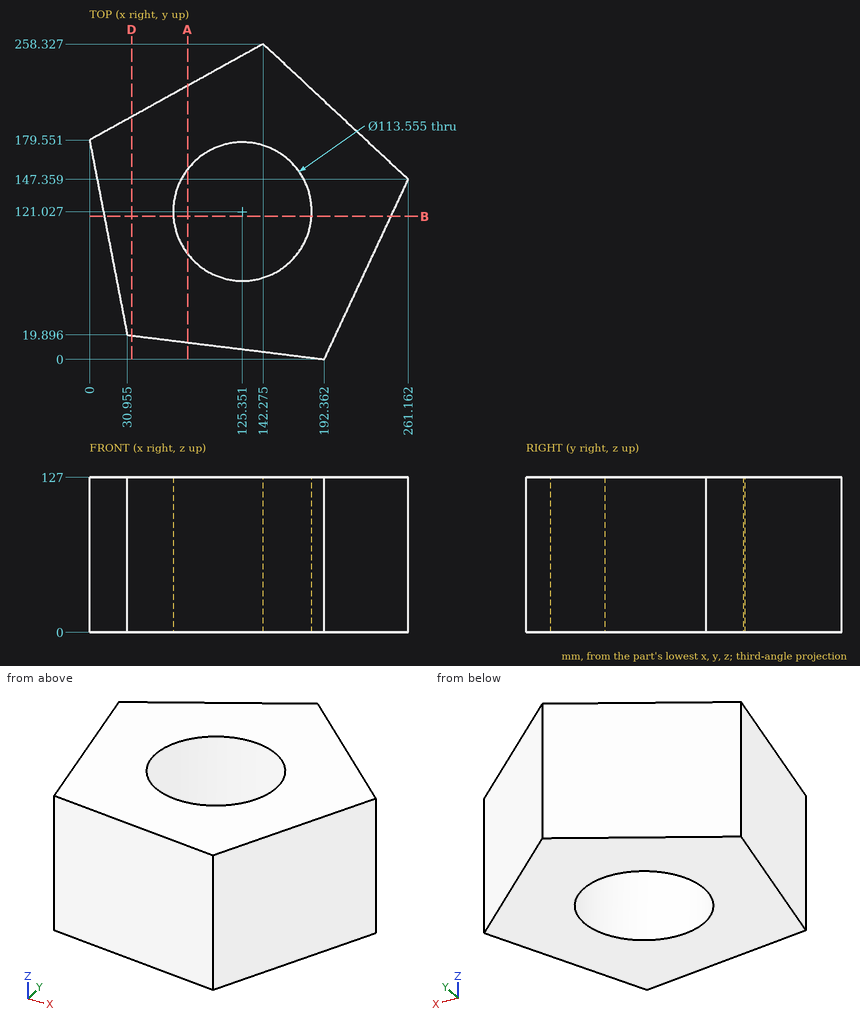
The figure shows three views and two pictorial views of one solid part (mm, origin at its lowest corner). Answer the questions. Give positions to 0.01 mm unless a question says otherwise; leave off trailing zeros. Order: outer loops, then holes, each group sorted by start corner. A loop starts at its lowest first (then second) coordinate and runs counter-clockwise, first axis right, second up. Notation, with made-up numbers: (28.25, 73.5) -> (38.25, 73.5) arc R8 ccw to (38.25, 84.5) -> close; hole circle Ø6 at (19, -24). An arc over 180 degrees is marked (long way). Answer as CSV lines item,"result". Start each with the question number.
Q1. A cutting plane is placed at D-D (x = 34.5). Determine the outline of the cut face in (y, z).
Q2. A cutting plane is placed at A-A (x = 80.5). Determine the outline of the cut face in (y, z).
Q3. Find the intervals of material crossed by L1, parallel to Y at x = 103, z = 109 (1 decimal); L2, parallel to Y at x = 76.5, z = 74 (1 decimal); L3, parallel to X at y = 110, z = 74 (1 decimal), in increasing order.
Q4. Given pin 1 (1 mm diameter, centred on x = 66.5, z = 43.5, fed in from +Y); pin 2 (8 mm diameter, centred on y = 93.5, z = 100, fed in from -X); pin 3 (6 mm diameter, centred on y = 100, z = 98.5, fed in from +X), each flat-ended and moving along its own axis, determine where each tip first touches the part or whether it passes through.
Q5. A cutting plane is placed at B-B (y = 117). Determine the outline of the cut face in (x, z) (1 decimal), then the cut area to 3 significant figures.
Results found:
1,outline,"(19.46, 0) -> (198.65, 0) -> (198.65, 127) -> (19.46, 127) -> close"
2,outline,"(13.79, 0) -> (86.21, 0) -> (86.21, 127) -> (13.79, 127) -> close; (155.84, 0) -> (224.12, 0) -> (224.12, 127) -> (155.84, 127) -> close"
3,L1,"11 to 68.8, 173.2 to 236.6"
3,L2,"14.3 to 92.1, 150 to 221.9"
3,L3,"13.5 to 69.7, 181 to 243.7"
4,pin 1,"y = 216.65"
4,pin 2,"x = 15.91"
4,pin 3,"x = 240.45"
5,outline,"(12.1, 0) -> (68.7, 0) -> (68.7, 127) -> (12.1, 127) -> close; (182, 0) -> (247, 0) -> (247, 127) -> (182, 127) -> close"
5,area,"15,400 mm2"
